For this review, take the finished solid that the model builds, in its own axes (mm). A direction names the side the tool comes from. Round coordinates to 2 decimals unless told otherwise and drop trailing zeros. Order: outer loops, then holes, each group sorted by start corner. A loop starts at its lowest first (then second) coordinate and runs counter-clockwise, first axis right, second up. Notation, with made-up numbers: M -26,-27.5 L -11,-27.5 A24 ccw -11,-2.5 Z; hole C 20.25,-12.75 d2. An arc over 180 degrees is marked long. Put each result on its own line as item: value.
from build123d import *

# Parameters (mm, degrees)
BOSS_EXTRUDE1_DEPTH = 152.4
SCALE1_SCALE        = 0.7
SKETCH2_W           = 99.568
SKETCH2_H           = 106.68
BOSS_EXTRUDE2_DEPTH = 17.78
SKETCH3_R           = 3.302
CUT_EXTRUDE1_DEPTH  = 0.254


with BuildPart() as part:
    # Sketch1 → Boss-Extrude1 (new body)
    with BuildSketch(Plane(origin=(0, 0, 0), x_dir=(1, 0, 0), z_dir=(0, 1, 0))):
        with BuildLine():
            Line((0, 0), (0, 56))
            Line((0, 56), (9.144, 56))
            Line((9.144, 56), (9.144, 61.08))
            ThreePointArc((9.144, 61.08), (10.722825004, 63.5214881), (9.652, 66.224613392))
            Line((9.652, 66.224613392), (9.652, 77.400613392))
            Line((9.652, 77.400613392), (45.72, 77.400613392))
            Line((45.72, 77.400613392), (45.72, 69.780613392))
            Line((45.72, 69.780613392), (96.52, 69.780613392))
            Line((96.52, 69.780613392), (96.52, 77.400613392))
            Line((96.52, 77.400613392), (132.588, 77.400613392))
            Line((132.588, 77.400613392), (132.588, 66.224613392))
            ThreePointArc((132.588, 66.224613392), (131.517174996, 63.5214881), (133.096, 61.08))
            Line((133.096, 61.08), (133.096, 56))
            Line((133.096, 56), (142.24, 56))
            Line((142.24, 56), (142.24, 0))
            Line((142.24, 0), (0, 0))
        make_face()
    extrude(amount=BOSS_EXTRUDE1_DEPTH)


with BuildPart() as part_1:
    # Scale1: scaled about (71.12, 76.2, -36.236599561)
    add(part.part.scale(SCALE1_SCALE).moved(Location((21.336, 22.86, -10.870979868))))

    # Sketch2 → Boss-Extrude2 (add)
    with BuildSketch(Plane.XY.offset(-10.870979868)):
        with Locations((71.12, 76.2)):
            Rectangle(SKETCH2_W, SKETCH2_H)
    extrude(amount=BOSS_EXTRUDE2_DEPTH)

    # Sketch3 → Cut-Extrude1 (cut)
    with BuildSketch(Plane.XZ.offset(-129.54)):
        with Locations(Location((71.12, -23.570979868, 0), (0, 0, 270))):
            Circle(SKETCH3_R)
    extrude(amount=CUT_EXTRUDE1_DEPTH, mode=Mode.SUBTRACT)


solid = part_1.part
(1) Draft analysis for pull direction Z (two halves, no side actions). For faces 1 (the face through (41, 75, -65.051)), 2 (the face through (70, 129.54, -30)), 3 (the face through (71, 129.286, -24)), state which applies: released by +Z, released by -Z, zero draft, split by the parting line, or undercut.
A:
face 1: released by -Z
face 2: zero draft
face 3: undercut
(2) Insertion check: pin 1 Ø5 at (x, y) = (119, 69) entering from -Z; pin 2 Ø6 at (y, z) = (107, -57.5) entering from +X; pin 3 Ø7.5 at (x, z) = (72, -24) entering from +Y; pin 4 Ø8.5 at (y, z) = (89, -60) entering from -X. Each pin has a flat end and moves straight along its axis. Give the tip position at first contact, or say it passes through.
A:
pin 1: stops at z = -50.07
pin 2: stops at x = 114.15
pin 3: stops at y = 129.54
pin 4: stops at x = 28.09
(3) To check wall thickness, follow L1, parallel to Z at x = 27.5, y = 98; L2, parallel to Z at x = 71, y = 129; L3, parallel to X at y = 97, z = -51.5. State the ranges of each line that lie inside material, in increasing order.
A:
L1: z = -50.07 to 6.91
L2: z = -59.72 to 6.91
L3: x = 27.74 to 114.5
(4) For faces 4 (the face through (24, 75, -50.071)), 5 (the face through (114.148, 75, -61)), 6 (the face through (53.34, 75, -62)), list the 3-axis set-ups (+Z, -Z, +X, -X, +Y, -Y) from which the entire face can be reached by the end or side of a thin tool; tool diameter is ignored.
A:
face 4: -Z, -X, +Y, -Y
face 5: -Z, +X, +Y, -Y
face 6: -Z, +Y, -Y
(5) Add section A-A on x = 71.12. Give the boundary of the cut face in (y, z), then the cut area to 3 significant figures.
A:
outline: M 22.86,-59.72 L 129.54,-59.72 L 129.54,-26.87 L 129.29,-26.87 L 129.29,-20.27 L 129.54,-20.27 L 129.54,6.91 L 22.86,6.91 Z
area: 7,110 mm2
(6) Add section B-B on y = 96. Give the boundary of the cut face in (x, z) (1 decimal), then the cut area to 3 significant figures.
A:
outline: M 21.3,-50.1 L 27.7,-50.1 L 27.7,-53.6 A2.2 cw 28.1,-57.2 L 28.1,-65.1 L 53.3,-65.1 L 53.3,-59.7 L 88.9,-59.7 L 88.9,-65.1 L 114.1,-65.1 L 114.1,-57.2 A2.2 cw 114.5,-53.6 L 114.5,-50.1 L 120.9,-50.1 L 120.9,6.9 L 21.3,6.9 Z
area: 6,770 mm2
(7) Add section C-C on x = 85. Give the boundary of the cut face in (y, z).
A:
outline: M 22.86,-59.72 L 129.54,-59.72 L 129.54,6.91 L 22.86,6.91 Z
